Geometry: final body of the model. Coordinates: model frame, mm. Coordinates: 2 decimals unless noted, no trailing zeros. Loops run counter-clockwise (first coordinate to the right, second up) from the corner with the lowest first, then second, coordinate; pieces in that order, holes last. Notation, with made-up numbers: (26, 13) - (74, 13) arc R20 ccw to (74, 50) - close; hole circle Ø2 at (-16, 11.25). An arc over 180 degrees is marked (long way). Write each question's results on one line, items separated by ' | '. Start each with the question number.
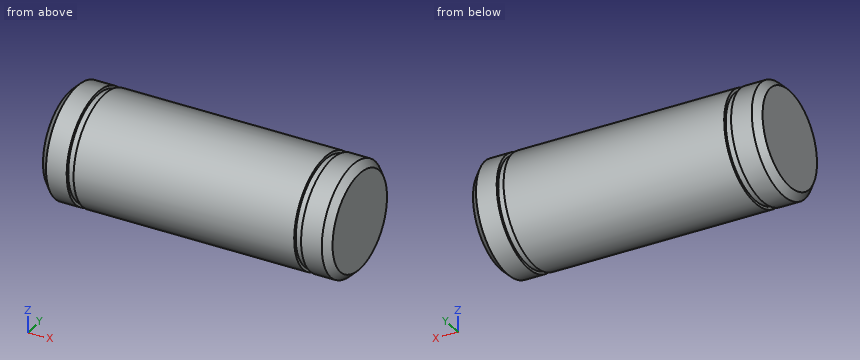
from build123d import *

# Parameters (mm, degrees)
SKETCH1_R           = 2
BOSS_EXTRUDE1_DEPTH = 10.5
CUT_EXTRUDE2_START  = -1
SKETCH2_R           = 2.498108329
SKETCH2_R_2         = 1.9
CUT_EXTRUDE2_DEPTH  = 0.25
CUT_EXTRUDE3_START  = -1.25
SKETCH3_R           = 2.5
SKETCH3_R_2         = 1.9
CUT_EXTRUDE3_DEPTH  = 0.25
CHAMFER1_SIZE       = 0.25


with BuildPart() as part:
    # Sketch1 → Boss-Extrude1 (new body)
    with BuildSketch(Plane(origin=(0, 0, 0), x_dir=(0, 0, -1), z_dir=(1, 0, 0))):
        with Locations(Location((0, 0, 0), (0, 0, 180))):
            Circle(SKETCH1_R)
    extrude(amount=BOSS_EXTRUDE1_DEPTH)

    # Sketch2 → Cut-Extrude2 (cut)
    with BuildSketch(Plane(origin=(10.5, 0, 0), x_dir=(0, 0, -1), z_dir=(1, 0, 0)).offset(CUT_EXTRUDE2_START)):
        Circle(SKETCH2_R)
        Circle(SKETCH2_R_2, mode=Mode.SUBTRACT)
    extrude(amount=-CUT_EXTRUDE2_DEPTH, mode=Mode.SUBTRACT)

    # Sketch3 → Cut-Extrude3 (cut)
    with BuildSketch(Plane.ZY.offset(CUT_EXTRUDE3_START)):
        Circle(SKETCH3_R)
        with Locations(Location((0, 0, 0), (0, 0, 180))):
            Circle(SKETCH3_R_2, mode=Mode.SUBTRACT)
    extrude(amount=CUT_EXTRUDE3_DEPTH, mode=Mode.SUBTRACT)

    # Chamfer1
    chamfer1_edges = [part.edges().sort_by_distance(p)[0] for p in [
        (0, 0, -2),
        (10.5, 0, -2),
    ]]
    chamfer(chamfer1_edges, length=CHAMFER1_SIZE)


solid = part.part
1) Pin query (flat end, axial travel): pin 1 Ø1.2 at (y, z) = (-1, 1) entering from -X. Return the tip coordinate at first contact, or that it passes through.
2) Section query A-A on x = 8.25. Output: boundary loops of the cut face in (y, z), and give its area (3 significant figures).
3) Material intervals for line 1 (Y direction, x = 4.75, z = -0.1); line 2 (Z direction, x = 3.5, y = -0.2); line 3 (Z direction, x = 3.5, y = -1.1), sorted ascending. Write a range as [from, to].
Returned:
1) pin 1: stops at x = 0
2) outline: circle Ø4 at (0, 0) | area: 12.6 mm²
3) line 1: y = [-2, 2] | line 2: z = [-1.99, 1.99] | line 3: z = [-1.67, 1.67]
